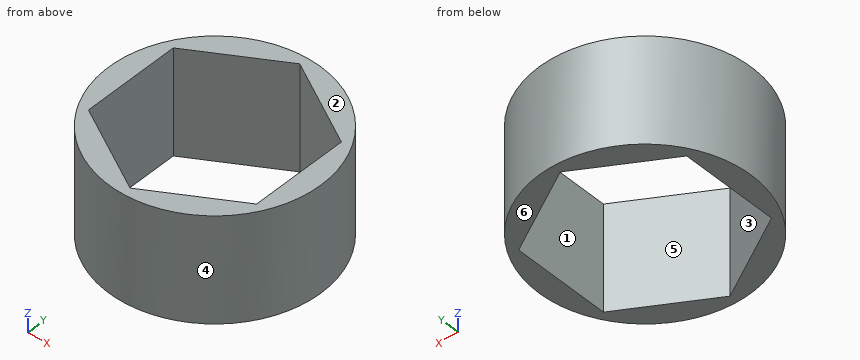
```python
from build123d import *

# Parameters (mm, degrees)
SKETCH1_R               = 12
SKETCH1_R_2             = 6.4
BOSS_EXTRUDE1_DEPTH     = 6
SKETCH1_4_R             = 6.4
CUT_EXTRUDE4_DEPTH      = 7
CUT_EXTRUDE4_DEPTH_BACK = 7


with BuildPart() as part:
    # Sketch1 → Boss-Extrude1 (new body, symmetric)
    with BuildSketch(Plane.XY):
        Circle(SKETCH1_R)
        Circle(SKETCH1_R_2, mode=Mode.SUBTRACT)
    extrude(amount=BOSS_EXTRUDE1_DEPTH, both=True)

    # Sketch1_4 → Cut-Extrude4 (cut, two sides)
    with BuildSketch(Plane.XY) as cut_extrude4_sk:
        Circle(SKETCH1_4_R)
        Polygon((-9.526279442, 5.5), (-9.526279442, -5.5), (0, -11), (9.526279442, -5.5), (9.526279442, 5.5), (0, 11), align=None)
        Circle(SKETCH1_4_R, mode=Mode.SUBTRACT)
    extrude(amount=CUT_EXTRUDE4_DEPTH, mode=Mode.SUBTRACT)
    extrude(cut_extrude4_sk.sketch, amount=-CUT_EXTRUDE4_DEPTH_BACK, mode=Mode.SUBTRACT)


solid = part.part
```
Design review of the part built by this model. Coordinates are the model's own, in mm. Face numbers are marked on the shaded views. A direction names the side the tool comes from. Coordinates: 2 decimals unless noted, no trailing zeros. Loops run counter-clockwise (first coordinate to the right, second up) from the corner with the lowest first, then second, coordinate; pieces in that order, holes last.
Q1. We need section C-C on z = 4. State the section outline as (x, y) points, and give its area (3 significant figures).
Reported:
outline: circle Ø24 at (0, 0); hole (-9.53, -5.5) - (0, -11) - (9.53, -5.5) - (9.53, 5.5) - (0, 11) - (-9.53, 5.5) - close
area: 138 mm2
Q2. For pin 1 (1 mm diameter, centred on y = 5.5, z = -1, fed in from -X); pin 2 (3 mm diameter, centred on y = 7.5, z = -1.5, fed in from +X); pin 3 (6 mm diameter, centred on x = 8, z = -1, fed in from +Y), all flat-tipped, find the tip position at first contact; note any pin that passes through.
Reported:
pin 1: stops at x = -10.91
pin 2: stops at x = 10.39
pin 3: stops at y = 10.91
Q3. To check wall thickness, follow line 1 (X direction, y = -7.25, z = 0.25); line 2 (X direction, y = 2, z = 4); line 3 (Y direction, x = -3, z = 1.5). State the ranges of each line that lie inside material, in increasing order.
Reported:
line 1: x = -9.56 to -6.5, 6.5 to 9.56
line 2: x = -11.83 to -9.53, 9.53 to 11.83
line 3: y = -11.62 to -9.27, 9.27 to 11.62
Q4. We need section B-B on x = 8.25. State the section outline as (y, z) points, and give its area (3 significant figures).
Reported:
outline: (-8.71, -6) - (-6.24, -6) - (-6.24, 6) - (-8.71, 6) - close; (6.24, -6) - (8.71, -6) - (8.71, 6) - (6.24, 6) - close
area: 59.5 mm2
Q5. The part is to be moulded in two halves that separate along Y. For the marked faces 1, 2, 3 and 4, say which applies: +Y half, -Y half, draft (parallel to the pull), parting line (faces both ways), or undercut.
Reported:
face 1: undercut
face 2: draft
face 3: undercut
face 4: parting line
Q6. We need section A-A on y = 0. State the section outline as (x, z) points.
Reported:
outline: (-12, -6) - (-9.53, -6) - (-9.53, 6) - (-12, 6) - close; (9.53, -6) - (12, -6) - (12, 6) - (9.53, 6) - close
Q7. Tool access review of the marked faces 5 and 6: name each direction out of +Z, -Z, +X, -X, +Y, -Y from which nothing blocks a thin tool from reaching the whole face with its end or side.
Reported:
face 5: +Z, -Z
face 6: -Z, +X, -X, +Y, -Y
